from build123d import *

# Parameters (mm, degrees)
F0_R     = 9.082794509
F1_DEPTH = 3.175
F2_SCALE = 0.8


# Not quite as in the source:
# - a feature names something its author has since deleted; it is built from what else it names


with BuildPart() as f1:
    # F0 (on Top) → F1 (new body)
    with BuildSketch(Plane.XY):
        with BuildLine():
            Line((190.1853488741, -177.0173265019), (349.6757983606, -156.6053567409))
            ThreePointArc((349.6757983606, -156.6053567409), (414.8838780797, -91.7557523294), (397.7330321915, -1.4041428346))
            Line((397.7330321915, -1.4041428346), (342.5045750448, 67.5291355358))
            add(Edge.make_bspline(
                [(329.4549969886, 114.1704269865), (331.5452640948, 111.8836468118), (336.0081220097, 107.0012205554), (339.0892090613, 95.2737066428), (342.2686372384, 79.5699362539), (342.4299296899, 71.3385709799), (342.5045750448, 67.5291355358)],
                knots=[0, 0, 0, 0, 0.2181778066, 0.4658239841, 0.7527859619, 1, 1, 1, 1], degree=3))
            add(Edge.make_bspline(
                [(329.4549969886, 114.1704269865), (326.548311382, 115.2426951096), (320.3423462083, 117.5320581607), (308.3194887471, 115.9577079905), (292.5774945842, 112.9732838027), (284.8943646943, 110.0150910055), (281.3386498949, 108.6460538997)],
                knots=[0, 0, 0, 0, 0.2181778066, 0.4658239841, 0.7527859619, 1, 1, 1, 1], degree=3))
            Line((281.3386498949, 108.6460538997), (196.6563418366, 133.7634989848))
            ThreePointArc((196.6563418366, 133.7634989848), (106.5159411756, 115.5351413614), (71.0829640293, 30.6701368923))
            Line((71.0829640293, 30.6701368923), (112.3931918139, -124.7239333526))
            Line((112.3931918139, -124.7239333526), (124.9610056376, -171.9994834736))
            Line((124.9610056376, -171.9994834736), (128.3971803048, -184.9251243198))
            Line((128.3971803048, -184.9251243198), (141.6635569768, -183.2272616556))
            Line((141.6635569768, -183.2272616556), (190.1853488741, -177.0173265019))
        make_face()
        with Locations((314.69919144, 47.0405749589)):
            Circle(F0_R, mode=Mode.SUBTRACT)
        with Locations((272.863497229, 75.1633380718)):
            Circle(F0_R, mode=Mode.SUBTRACT)
        with BuildLine():
            ThreePointArc((112.3931918139, -124.7239333526), (93.1968044826, -155.1354338039), (124.9610056376, -171.9994834736))
            Line((124.9610056376, -171.9994834736), (112.3931918139, -124.7239333526))
        make_face()
        with BuildLine():
            ThreePointArc((141.6635569768, -183.2272616556), (169.2714467636, -206.2742802869), (190.1853488741, -177.0173265019))
            Line((190.1853488741, -177.0173265019), (141.6635569768, -183.2272616556))
        make_face()
        with BuildLine():
            Line((120.3224166543, -196.9372207683), (128.3971803048, -184.9251243198))
            Line((128.3971803048, -184.9251243198), (124.9610056376, -171.9994834736))
            Line((124.9610056376, -171.9994834736), (115.7260780635, -198.4687475134))
            ThreePointArc((115.7260780635, -198.4687475134), (117.6479584787, -196.5736854806), (120.3224166543, -196.9372207683))
        make_face()
        with BuildLine():
            Line((120.6394586436, -201.7716170066), (141.6635569768, -183.2272616556))
            Line((141.6635569768, -183.2272616556), (128.3971803048, -184.9251243198))
            Line((128.3971803048, -184.9251243198), (120.3224166543, -196.9372207683))
            ThreePointArc((120.3224166543, -196.9372207683), (121.6687259476, -199.2765231696), (120.6394586436, -201.7716170066))
        make_face()
        with BuildLine():
            ThreePointArc((116.9081491924, -202.0163180432), (118.8155291594, -202.53021243), (120.6394586436, -201.7716170066))
            ThreePointArc((120.6394586436, -201.7716170066), (121.6687259476, -199.2765231696), (120.3224166543, -196.9372207683))
            Line((120.3224166543, -196.9372207683), (116.9081491924, -202.0163180432))
        make_face()
        with BuildLine():
            Line((116.9081491924, -202.0163180432), (120.3224166543, -196.9372207683))
            ThreePointArc((120.3224166543, -196.9372207683), (117.6479584787, -196.5736854806), (115.7260780635, -198.4687475134))
            ThreePointArc((115.7260780635, -198.4687475134), (115.7121989982, -200.4440938504), (116.9081491924, -202.0163180432))
        make_face()
    extrude(amount=F1_DEPTH)


with BuildPart() as f1_1:
    # F2: moved
    add(f1.part.scale(F2_SCALE).moved(Location((51.3425254966, 2.2402065434, 0))))


solid = f1_1.part
Geometry check sheet. Reference: the model listing, model coordinates, mm. A direction names the side the tool comes from. Give positions to 0.01 mm unless a question says otherwise; leave off trailing zeros. Order: outer loops, then holes, each group sorted by start corner. A loop starts at its lowest first (then second) coordinate and runs counter-clockwise, first axis right, second up. Notation, with made-up numbers: M 48,-14 L 98,-14 A28 cw 98,9 Z; hole C 49.5,38 d4. An arc over 180 degrees is marked long. Use a Markdown table: item, result.
Item 1: Section check A-A (z = 1.7). State how many separate pieces and enclosed holes the cut face has, and give its area (3 significant figures).
Answers follow:
| item | result |
|---|---|
| separate pieces | 1 |
| enclosed holes | 2 |
| area | 55,600 mm2 |
Item 2: Draft check along Y on faces 1 (the flat face through (245, -23, 0)), 2 (the cylindrical face through (262.374, 62.69, 1.252)), 3 (the flat face through (347.75, 28.3, 1.25)). Enter one of: +Y half, -Y half, draft (parallel to the pull), parting line (faces both ways), or undercut.
Answers follow:
| item | result |
|---|---|
| face 1 | draft |
| face 2 | undercut |
| face 3 | +Y half |
Item 3: Section check B-B (y = -47). Record the cut outline in (x, z).
Answers follow:
| item | result |
|---|---|
| outline | M 127.82,0 L 386.76,0 L 386.76,2.54 L 127.82,2.54 Z |
Item 4: Tool access check on faces 4 (the flat face through (156.15, -151.86, 1.25)), 5 (the flat face through (124.5, -34.5, 1.3)), 6 (the flat face through (243.015, 99.063, 1.252)), 7 (the flat face through (245, -23, 2.54)). Record the directions out of +Z, -Z, +X, -X, +Y, -Y that give a thin tool (end or side, any length) a straight path to the whole face; none if there is none.
Answers follow:
| item | result |
|---|---|
| face 4 | +Z, -Z, -Y |
| face 5 | +Z, -Z, -X |
| face 6 | +Z, -Z, +Y |
| face 7 | +Z, +X, -X, +Y, -Y |
Item 5: Depth check by flat-ended pin: P1, Ø1, axis at x = 235, z = 0.5, coming from the -Y side (3 decimals); P2, Ø1, axis at x = 192, z = 2, coming from the -Y side. Enter the tip coordinate at first touch or a pass-through.
Answers follow:
| item | result |
|---|---|
| P1 | stops at y = -135.405 |
| P2 | stops at y = -161.56 |
Item 6: Section check C-C (x = 257). Record the cut outline in (y, z), and give its area (3 significant figures).
Answers follow:
| item | result |
|---|---|
| outline | M -132.53,0 L 94.92,0 L 94.92,2.54 L -132.53,2.54 Z |
| area | 578 mm2 |
Item 7: Material ranges on line 1 along X through (y, z) = (-145, 0.7); line 2 along X through (y, z) = (68, 1.5); line 3 along Y through (x, z) = (142, 2), recorded low to high.
Answers follow:
| item | result |
|---|---|
| line 1 | x = 147.95 to 163.93, 164.72 to 203.82 |
| line 2 | x = 115.62 to 265.04, 274.23 to 324.54 |
| line 3 | y = -136.24 to 98.76 |
